from build123d import *

# Parameters (mm, degrees)
BOSS_EXTRUDE1_DEPTH = 6
SKETCH2_W           = 2
SKETCH2_H           = 24
BOSS_EXTRUDE2_DEPTH = 4


with BuildPart() as part:
    # Sketch1 → Boss-Extrude1 (new, symmetric)
    with BuildSketch(Plane(origin=(0, 0, 0), x_dir=(0, 0, -1), z_dir=(1, 0, 0))):
        Polygon((-2.5, -27.858843537), (-2.5, 2.141156463), (-17.5, 2.141156463), (-17.5, 30.641156463), (-15.5, 29.641156463), (-15.5, 5.641156463), (15.5, 5.641156463), (15.5, 29.641156463), (17.5, 30.641156463), (17.5, 2.141156463), (2.5, 2.141156463), (2.5, -27.858843537), align=None)
    extrude(amount=BOSS_EXTRUDE1_DEPTH, both=True)

    # Sketch2 → Boss-Extrude2 (add)
    with BuildSketch(Plane(origin=(0, 0, 15.5), x_dir=(-1, 0, 0), z_dir=(0, 0, -1))):
        with Locations((-5, 17.641156463)):
            Rectangle(SKETCH2_W, SKETCH2_H)
    boss_extrude2 = extrude(amount=BOSS_EXTRUDE2_DEPTH)

    # Mirror1: Boss-Extrude2 across plane
    add(boss_extrude2.mirror(Plane(origin=(0, 0, 0), x_dir=(1, 0, 0), z_dir=(0, 0, -1))))


solid = part.part
Geometry check sheet. Reference: the model listing, model coordinates, mm. A direction names the side the tool comes from. Round coordinates to 2 decimals unless told otherwise and drop trailing zeros. Order: outer loops, then holes, each group sorted by start corner. A loop starts at its lowest first (then second) coordinate and runs counter-clockwise, first axis right, second up. Notation, with made-up numbers: (78, 34) -> (133, 34) arc R33 cw to (133, 73) -> close; hole circle Ø6 at (14.25, 27). An arc over 180 degrees is marked (long way). Use one line per item in the form item = value.
1. Cross-section at D-D, the plane z = 7.5. Enter the section's corners in (x, y).
Working result:
outline = (-6, 2.14) -> (6, 2.14) -> (6, 5.64) -> (-6, 5.64) -> close
2. Mould release check, pull along Z, two halves, no side actions. Record for faces 1 (the face through (0.084, 30.148, 16.514)), 2 (the face through (0, -13, 2.5)), 3 (the face through (0, -27.859, 0)), 4 (the face through (0, -13, -2.5)): pulls with the +Z half, pulls with the -Z half, needs draft (parallel to the pull), parting line crosses it, or undercut.
Working result:
face_1 = undercut
face_2 = pulls with the +Z half
face_3 = needs draft
face_4 = pulls with the -Z half
3. Set-up check for faces 5 (the face through (0, 2.141, -10)), 6 (the face through (5, 18, 11.5)), 7 (the face through (-1, 17, -15.5)), 8 (the face through (0, 2.141, 10)): record each of +Z, -Z, +X, -X, +Y, -Y from which the full face is reachable in a straight line by a thin tool's end or side.
Working result:
face_5 = -Z, +X, -X, -Y
face_6 = +X, -X, +Y
face_7 = -X, +Y
face_8 = +Z, +X, -X, -Y
4. Cross-section at B-B, the plane x = -0.25. Enter the section's corners in (y, z), plus the area to 4 significant figures.
Working result:
outline = (-27.86, -2.5) -> (2.14, -2.5) -> (2.14, -17.5) -> (30.64, -17.5) -> (29.64, -15.5) -> (5.64, -15.5) -> (5.64, 15.5) -> (29.64, 15.5) -> (30.64, 17.5) -> (2.14, 17.5) -> (2.14, 2.5) -> (-27.86, 2.5) -> close
area = 370.5 mm^2
5. Cross-section at A-A, the plane y = 16. Enter the section's corners in (x, z), plus the area to 3 significant figures.
Working result:
outline = (-6, -17.5) -> (6, -17.5) -> (6, -11.5) -> (4, -11.5) -> (4, -15.5) -> (-6, -15.5) -> close; (-6, 15.5) -> (4, 15.5) -> (4, 11.5) -> (6, 11.5) -> (6, 17.5) -> (-6, 17.5) -> close
area = 64.0 mm^2
6. Cross-section at C-C, the plane y = -18. Enter the section's corners in (x, z).
Working result:
outline = (-6, -2.5) -> (6, -2.5) -> (6, 2.5) -> (-6, 2.5) -> close
7. Scan lines: line 1 along Z through (x, y) = (2.25, 16); line 2 along Z through (x, y) = (5, 7); line 3 along Z through (x, y) = (-0.75, -23). Record each from-to range of solid material in increasing order. Write a range as from..to.
Working result:
line_1 = -17.5..-15.5, 15.5..17.5
line_2 = -17.5..-11.5, 11.5..17.5
line_3 = -2.5..2.5
8. Go/stop test with flat-tipped pins: pin 1 (3.5 mm diameter, centred on x = -2, y = -20, fed in from +Z); pin 2 (1.6 mm diameter, centred on x = 4.5, z = 14, fed in from +Y); pin 3 (3.5 mm diameter, centred on x = 1, y = -17.5, fed in from -Z). Record where each tip stops, or that it passes through.
Working result:
pin_1 = 2.5
pin_2 = 29.64
pin_3 = -2.5
